Could you check a few things on this drawing? It's one solid part, dimensions in mm from its lowest x, y, z. A direction names the side the tool comes from. Coordinates: 2 decimals unless noted, no trailing zeros. Write each loop counter-clockwise with the first axis right and the second up, starting at its lowest first coordinate (ties: lowest second). Pieces come first, ordered by that corner, then holes.
Item 1: I'm going to push flat-ended pins straight in: P1, Ø3, axis at y = 2, z = 11.5, coming from the +X side; P2, Ø2, axis at x = 5, y = 2, coming from the +Z side (1 decimal); P3, Ø4, axis at x = 16, y = 7, coming from the -Z side. Where does each tip first touch, or does it pass through?
Item 2: Please list where these lines run through material, in increasing order: line 1 (Y direction, x = 1, z = 7) (1 decimal); line 2 (Y direction, x = 5.5, z = 16.5); line 3 (Z direction, x = 9.5, y = 1.25) (1 decimal).
Item 3: I want a section at A-A (y = 6.75). Please give me the cut outline in (x, z) (1 decimal).
Item 4: If we mould it in two halves opening along Y, with no side actions, what happens to the marked faces 3, 4 and 5? For each: pulls with the +Y half, pulls with the -Y half, needs draft (parallel to the pull), parting line crosses it, or undercut.
Item 5: I want a section at B-B (y = 10.25). Please give me the cut outline in (x, z) (1 decimal).
Item 6: For the marked faces 1 and 2, which set-ups out of +Z, -Z, +X, -X, +Y, -Y let a thin tool reach every point of the face, with its end or its side?
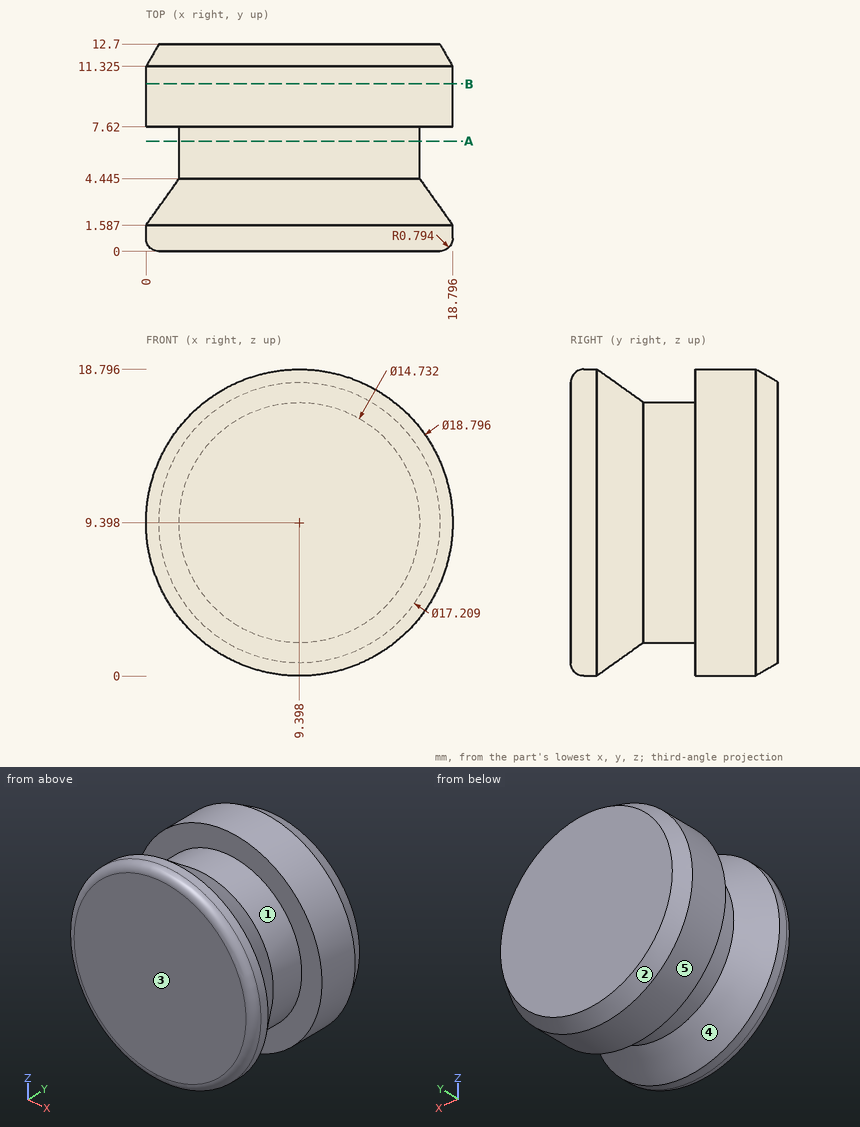
Answer:
1. P1: stops at x = 18.77
1. P2: stops at z = 18.1
1. P3: stops at z = 1.26
2. line 1: y = 0 to 2.5, 7.6 to 12.5
2. line 2: y = 0 to 3.41, 7.62 to 12.7
2. line 3: z = 0 to 18.8
3. outline: circle Ø14.7 at (9.4, 9.4)
4. face 3: pulls with the -Y half
4. face 4: undercut
4. face 5: needs draft
5. outline: circle Ø18.8 at (9.4, 9.4)
6. face 1: none
6. face 2: +Y
